Autodesk Inventor part; units mm, degrees
ref_plane "YZ Plane" through (0, 0, 0) normal (1, 0, 0) x (0, 1, 0)
ref_plane "XZ Plane" through (0, 0, 0) normal (0, 1, 0) x (-1, 0, 0)
ref_plane "XY Plane" through (0, 0, 0) normal (0, 0, 1) x (1, 0, 0)
sketch "Boceto1" plane through (0, 0, 0) normal (0, 0, 1) x (1, 0, 0)
  line L0 (0, 340) -> (400, 340)
  line L1 (400, 340) -> (400, 0)
  line L2 (70, 0) -> (70, 56.12)
  line L3 (0, 340) -> (0, 126)
  line L4 (0, 126) -> (70, 56.12)
  line L5 (0, 126) -> (0, 340)
  line L6 (70, 0) -> (400, 0)
  point P0 (0, 0)
  dimension "d0" = 340
  dimension "d1" = 400
  dimension "d2" = 70
  dimension "d3" = 56.12
  dimension "d4" = 214
extrude "Extrusión1" add sketch "Boceto1" along normal blind 530
properties part number "caja area de trabajo"
Verification items for the finished model (mm, model axes). A direction names the side the tool comes from. Coordinates: 2 decimals unless noted, no trailing zeros. Order: outer loops, then holes, each group sorted by start corner. A loop starts at its lowest first (then second) coordinate and runs counter-clockwise, first axis right, second up.
1. Go/stop test with flat-tipped pins: pin 1 Ø17 at (y, z) = (30.5, 333.5) entering from -X; pin 2 Ø5 at (y, z) = (86.5, 121) entering from -X. Record where each tip stops, or that it passes through.
Results found:
pin 1: stops at x = 70
pin 2: stops at x = 37.06
2. Set-up check for faces 1 (the face through (70, 28, 261)), 2 (the face through (197, 172, 530)): record each of +Z, -Z, +X, -X, +Y, -Y from which the full face is reachable in a straight line by a thin tool's end or side.
Results found:
face 1: +Z, -Z, -X, -Y
face 2: +Z, +X, -X, +Y, -Y
3. Scan lines: line 1 (X direction, y = 55, z = 318); line 2 (X direction, y = 102.5, z = 389.5); line 3 (Y direction, x = 67, z = 468). Record each from-to range of solid material in increasing order.
Results found:
line 1: x = 70 to 400
line 2: x = 23.54 to 400
line 3: y = 59.11 to 340
4. Sectioned sample at C-C, the plane y = 33. Record the cut outline in (x, z), and give its area (3 significant figures).
Results found:
outline: (70, 0) - (400, 0) - (400, 530) - (70, 530) - close
area: 175,000 mm2
5. Sectioned sample at B-B, the plane x = 52.5. Record the cut outline in (y, z).
Results found:
outline: (73.59, 0) - (340, 0) - (340, 530) - (73.59, 530) - close
6. Sectioned sample at A-A, the plane z = 204.5. Record the cut outline in (x, y), and give its area (3 significant figures).
Results found:
outline: (0, 126) - (70, 56.12) - (70, 0) - (400, 0) - (400, 340) - (0, 340) - close
area: 130,000 mm2
